from build123d import *

# Parameters (mm, degrees)
SKETCH_1_R          = 1.6
EXTRUDE_1_DEPTH     = 2
CUT_EXTRUDE_3_DEPTH = 169.328378846
CUT_EXTRUDE_4_DEPTH = 169.328378846
FILLET_2_R          = 5


with BuildPart() as part:
    # 草图1 → 凸台-拉伸1 (new body)
    with BuildSketch(Plane(origin=(0, 0, 0), x_dir=(1, 0, 0), z_dir=(0, 1, 0))):
        Polygon((-121.25, 83.825), (-121.25, -83.825), (-65, -83.825), (-65, -98.825), (-25, -98.825), (-25, -83.825), (25, -83.825), (25, -98.825), (65, -98.825), (65, -83.825), (121.25, -83.825), (121.25, -20), (136.25, -20), (136.25, 20), (121.25, 20), (121.25, 83.825), (65, 83.825), (65, 98.825), (25, 98.825), (25, 83.825), (-25, 83.825), (-25, 98.825), (-65, 98.825), (-65, 83.825), align=None)
        with Locations(Location((-30, -91.325, 0), (0, 0, 270))):
            Circle(SKETCH_1_R, mode=Mode.SUBTRACT)
        with Locations(Location((-60, -91.325, 0), (0, 0, 270))):
            Circle(SKETCH_1_R, mode=Mode.SUBTRACT)
        with Locations(Location((-30, 91.325, 0), (0, 0, 270))):
            Circle(SKETCH_1_R, mode=Mode.SUBTRACT)
        with Locations(Location((-60, 91.325, 0), (0, 0, 270))):
            Circle(SKETCH_1_R, mode=Mode.SUBTRACT)
        with Locations(Location((60, -91.325, 0), (0, 0, 270))):
            Circle(SKETCH_1_R, mode=Mode.SUBTRACT)
        with Locations(Location((30, -91.325, 0), (0, 0, 270))):
            Circle(SKETCH_1_R, mode=Mode.SUBTRACT)
        with Locations(Location((60, 91.325, 0), (0, 0, 270))):
            Circle(SKETCH_1_R, mode=Mode.SUBTRACT)
        with Locations(Location((30, 91.325, 0), (0, 0, 270))):
            Circle(SKETCH_1_R, mode=Mode.SUBTRACT)
        with Locations(Location((128.75, 15, 0), (0, 0, 270))):
            Circle(SKETCH_1_R, mode=Mode.SUBTRACT)
        with Locations(Location((128.75, -15, 0), (0, 0, 270))):
            Circle(SKETCH_1_R, mode=Mode.SUBTRACT)
    extrude(amount=EXTRUDE_1_DEPTH)

    # 草图4 → 切除-拉伸3 (cut, through all)
    with BuildSketch(Plane(origin=(0, 2, 0), x_dir=(1, 0, 0), z_dir=(0, 1, 0))):
        with BuildLine():
            Line((-92.15, 64.425), (-92.15, 19.4))
            ThreePointArc((-92.15, 19.4), (-101.85, 9.7), (-111.55, 19.4))
            Line((-111.55, 19.4), (-111.55, 64.425))
            ThreePointArc((-111.55, 64.425), (-101.85, 74.125), (-92.15, 64.425))
        make_face()
        with BuildLine():
            Line((-63.05, 64.425), (-63.05, 19.4))
            ThreePointArc((-63.05, 19.4), (-72.75, 9.7), (-82.45, 19.4))
            Line((-82.45, 19.4), (-82.45, 64.425))
            ThreePointArc((-82.45, 64.425), (-72.75, 74.125), (-63.05, 64.425))
        make_face()
        with BuildLine():
            Line((-33.95, 64.425), (-33.95, 19.4))
            ThreePointArc((-33.95, 19.4), (-43.65, 9.7), (-53.35, 19.4))
            Line((-53.35, 19.4), (-53.35, 64.425))
            ThreePointArc((-53.35, 64.425), (-43.65, 74.125), (-33.95, 64.425))
        make_face()
        with BuildLine():
            Line((-4.85, 64.425), (-4.85, 19.4))
            ThreePointArc((-4.85, 19.4), (-14.55, 9.7), (-24.25, 19.4))
            Line((-24.25, 19.4), (-24.25, 64.425))
            ThreePointArc((-24.25, 64.425), (-14.55, 74.125), (-4.85, 64.425))
        make_face()
        with BuildLine():
            Line((24.25, 64.425), (24.25, 19.4))
            ThreePointArc((24.25, 19.4), (14.55, 9.7), (4.85, 19.4))
            Line((4.85, 19.4), (4.85, 64.425))
            ThreePointArc((4.85, 64.425), (14.55, 74.125), (24.25, 64.425))
        make_face()
        with BuildLine():
            Line((53.35, 64.425), (53.35, 19.4))
            ThreePointArc((53.35, 19.4), (43.65, 9.7), (33.95, 19.4))
            Line((33.95, 19.4), (33.95, 64.425))
            ThreePointArc((33.95, 64.425), (43.65, 74.125), (53.35, 64.425))
        make_face()
        with BuildLine():
            Line((82.45, 64.425), (82.45, 19.4))
            ThreePointArc((82.45, 19.4), (72.75, 9.7), (63.05, 19.4))
            Line((63.05, 19.4), (63.05, 64.425))
            ThreePointArc((63.05, 64.425), (72.75, 74.125), (82.45, 64.425))
        make_face()
        with BuildLine():
            Line((111.55, 64.425), (111.55, 19.4))
            ThreePointArc((111.55, 19.4), (101.85, 9.7), (92.15, 19.4))
            Line((92.15, 19.4), (92.15, 64.425))
            ThreePointArc((92.15, 64.425), (101.85, 74.125), (111.55, 64.425))
        make_face()
        with BuildLine():
            Line((111.55, -64.425), (111.55, -19.4))
            ThreePointArc((111.55, -19.4), (101.85, -9.7), (92.15, -19.4))
            Line((92.15, -19.4), (92.15, -64.425))
            ThreePointArc((92.15, -64.425), (101.85, -74.125), (111.55, -64.425))
        make_face()
        with BuildLine():
            Line((82.45, -64.425), (82.45, -19.4))
            ThreePointArc((82.45, -19.4), (72.75, -9.7), (63.05, -19.4))
            Line((63.05, -19.4), (63.05, -64.425))
            ThreePointArc((63.05, -64.425), (72.75, -74.125), (82.45, -64.425))
        make_face()
        with BuildLine():
            Line((53.35, -64.425), (53.35, -19.4))
            ThreePointArc((53.35, -19.4), (43.65, -9.7), (33.95, -19.4))
            Line((33.95, -19.4), (33.95, -64.425))
            ThreePointArc((33.95, -64.425), (43.65, -74.125), (53.35, -64.425))
        make_face()
        with BuildLine():
            Line((24.25, -64.425), (24.25, -19.4))
            ThreePointArc((24.25, -19.4), (14.55, -9.7), (4.85, -19.4))
            Line((4.85, -19.4), (4.85, -64.425))
            ThreePointArc((4.85, -64.425), (14.55, -74.125), (24.25, -64.425))
        make_face()
        with BuildLine():
            Line((-4.85, -64.425), (-4.85, -19.4))
            ThreePointArc((-4.85, -19.4), (-14.55, -9.7), (-24.25, -19.4))
            Line((-24.25, -19.4), (-24.25, -64.425))
            ThreePointArc((-24.25, -64.425), (-14.55, -74.125), (-4.85, -64.425))
        make_face()
        with BuildLine():
            Line((-33.95, -64.425), (-33.95, -19.4))
            ThreePointArc((-33.95, -19.4), (-43.65, -9.7), (-53.35, -19.4))
            Line((-53.35, -19.4), (-53.35, -64.425))
            ThreePointArc((-53.35, -64.425), (-43.65, -74.125), (-33.95, -64.425))
        make_face()
        with BuildLine():
            Line((-63.05, -64.425), (-63.05, -19.4))
            ThreePointArc((-63.05, -19.4), (-72.75, -9.7), (-82.45, -19.4))
            Line((-82.45, -19.4), (-82.45, -64.425))
            ThreePointArc((-82.45, -64.425), (-72.75, -74.125), (-63.05, -64.425))
        make_face()
        with BuildLine():
            Line((-92.15, -64.425), (-92.15, -19.4))
            ThreePointArc((-92.15, -19.4), (-101.85, -9.7), (-111.55, -19.4))
            Line((-111.55, -19.4), (-111.55, -64.425))
            ThreePointArc((-111.55, -64.425), (-101.85, -74.125), (-92.15, -64.425))
        make_face()
    extrude(amount=-CUT_EXTRUDE_3_DEPTH, mode=Mode.SUBTRACT)

    # 草图5 → 切除-拉伸4 (cut, through all)
    with BuildSketch(Plane(origin=(0, 2, 0), x_dir=(1, 0, 0), z_dir=(0, 1, 0))):
        Polygon((-65, 83.825), (-65, 80.825), (-120.25, 80.825), (-120.25, -80.825), (-65, -80.825), (-65, -83.825), (-121.25, -83.825), (-121.25, 83.825), align=None)
        Polygon((65, -83.825), (65, -82.825), (120.25, -82.825), (120.25, -20), (121.25, -20), (121.25, -83.825), align=None)
        Polygon((121.25, 20), (120.25, 20), (120.25, 82.825), (65, 82.825), (65, 83.825), (121.25, 83.825), align=None)
    extrude(amount=-CUT_EXTRUDE_4_DEPTH, mode=Mode.SUBTRACT)

    # 圆角2
    fillet_2_edges = [part.edges().sort_by_distance(p)[0] for p in [
        (-65, 1, -80.825),
        (-120.25, 1, -80.825),
        (-120.25, 1, 80.825),
        (-65, 1, 80.825),
        (65, 1, 82.825),
        (120.25, 1, 82.825),
        (120.25, 1, 20),
        (120.25, 1, -20),
        (120.25, 1, -82.825),
        (65, 1, -82.825),
        (-65, 1, -98.825),
        (-25, 1, -98.825),
        (-25, 1, -83.825),
        (25, 1, -83.825),
        (25, 1, -98.825),
        (65, 1, -98.825),
        (136.25, 1, -20),
        (136.25, 1, 20),
        (65, 1, 98.825),
        (25, 1, 98.825),
        (25, 1, 83.825),
        (-25, 1, 83.825),
        (-25, 1, 98.825),
        (-65, 1, 98.825),
    ]]
    fillet(fillet_2_edges, radius=FILLET_2_R)


solid = part.part
CAD build for the part. Positions are in the model's coordinates, mm. A direction names the side the tool comes from. Give positions to 0.01 mm unless a question says otherwise; leave off trailing zeros. Loops run counter-clockwise (first coordinate to the right, second up) from the corner with the lowest first, then second, coordinate; pieces in that order, holes last. Notation, with made-up numbers: M 20,-30 L 26,-30 A11 cw 26,-24 Z; hole C 60,-12.75 d1. An arc over 180 degrees is marked long. Answer in a Markdown table with one row per item. Add a question column.
Item 1: Band-saw the part on A-A on x = -101.85. Give the cut face in (y, z) (3 decimals).
Item 2: Tool access for faces 5 (the face through (66.426, 0.986, -84.329)), 6 (the face through (-23.574, 1.014, -85.329)), 7 (the face through (-43.863, 1.014, -74.123)): list every direction of +Z, -Z, +X, -X, +Y, -Y with a clear straight run to the whole face (end or side of a thin tool).
Item 3: Drop flat-ended pins along their axis: P1, Ø5, axis at x = 8, z = -49.5, coming from the -Y side; P2, Ø1, axis at y = 1, z = -91, coming from the +X side; P3, Ø1, axis at y = 1, z = 52, coming from the +X side; P4, Ø0.6, axis at x = -10, y = 0.5, coming from the +Z side (3 decimals). Give the stop position or say it passes through.
Item 4: Band-saw the part on B-B on z = 60.5. Give the number of separate pieces and of enclosed holes in the cut face, then the cut area to 3 significant figures.
Item 5: Band-saw the part on C-C on x = -14.55. Give the cut face in (y, z) (3 decimals).
Item 6: Probe probe 1 along Z at (x, y) = (128.75, 1); probe 2 along Z at (x, y) = (76, 0.5) (3 decimals); probe 3 along Z at (x, y) = (-89, 0.9) (3 decimals). List the from-to ranges inside material, lowest first.
Item 7: Mould opens along Z. For faces 1 (the face through (-14.763, 1.014, 74.123)), 2 (the face through (72.963, 1.014, -9.702)), 3 (the face through (-118.746, 0.986, 79.399)), 4 (the face through (121.68, 0.99, -21.5)) say: +Z half, -Z half, draft (parallel to the pull), parting line (faces both ways), or undercut.
Reply:
| question | item | result |
|---|---|---|
| 1 | outline | M 0,-80.825 L 2,-80.825 L 2,-74.125 L 0,-74.125 Z; M 0,-9.7 L 2,-9.7 L 2,9.7 L 0,9.7 Z; M 0,74.125 L 2,74.125 L 2,80.825 L 0,80.825 Z |
| 2 | face 5 | -Z, +X, +Y, -Y |
| 2 | face 6 | -Z, +Y, -Y |
| 2 | face 7 | +Y, -Y |
| 3 | P1 | passes through |
| 3 | P2 | stops at x = 65 |
| 3 | P3 | stops at x = 120.25 |
| 3 | P4 | stops at z = 83.825 |
| 4 | separate pieces | 9 |
| 4 | enclosed holes | 0 |
| 4 | area | 171 mm^2 |
| 5 | outline | M 0,-83.825 L 2,-83.825 L 2,-74.125 L 0,-74.125 Z; M 0,-9.7 L 2,-9.7 L 2,9.7 L 0,9.7 Z; M 0,74.125 L 2,74.125 L 2,83.825 L 0,83.825 Z |
| 6 | probe 1 | z = -20 to -16.6, -13.4 to 13.4, 16.6 to 20 |
| 6 | probe 2 | z = -82.825 to -73.564, -10.261 to 10.261, 73.564 to 82.825 |
| 6 | probe 3 | z = -80.825 to 80.825 |
| 7 | face 1 | undercut |
| 7 | face 2 | undercut |
| 7 | face 3 | +Z half |
| 7 | face 4 | -Z half |
